Read the model definition and answer for the solid it produces. Units are mm, in the model's axes. Give positions to 0.01 mm unless a question says otherwise; leave off trailing zeros. Order: outer loops, then holes, each group sorted by start corner. A loop starts at its lowest first (then second) coordinate and runs counter-clockwise, first axis right, second up. Notation, with made-up numbers: (-9.75, 4.5) - (45.25, 4.5) arc R11 ccw to (45.25, 21.5) - close; hole circle Ø11 at (5.5, -2). An arc over 180 degrees is marked (long way). Write each question's results on one line, items separated by ' | '.
from build123d import *

# Parameters (mm, degrees)
BOSS_EXTRUDE1_DEPTH = 6.35
FILLET1_R           = 19.05
SKETCH4_R           = 10.5
SKETCH4_R_2         = 6.4
SKETCH4_R_3         = 1.5
CUT_EXTRUDE1_DEPTH  = 7.35


with BuildPart() as part:
    # Sketch3 → Boss-Extrude1 (new body)
    with BuildSketch(Plane.XY):
        Polygon((-152.4, 25.4), (50.8, 25.4), (175.63877155, -62.0130489), (-27.56122845, -62.0130489), align=None)
    extrude(amount=BOSS_EXTRUDE1_DEPTH)

    # Fillet1
    fillet1_edges = [part.edges().sort_by_distance(p)[0] for p in [
        (-152.4, 25.4, 3.175),
        (50.8, 25.4, 3.175),
        (175.63877155, -62.0130489, 3.175),
        (-27.56122845, -62.0130489, 3.175),
    ]]
    fillet(fillet1_edges, radius=FILLET1_R)

    # Sketch4 → Cut-Extrude1 (cut, through all)
    with BuildSketch(Plane.XY.offset(6.35)):
        with Locations((-91.981119015, 6.35)):
            Circle(SKETCH4_R)
        with Locations((38.393558072, 0)):
            Circle(SKETCH4_R_2)
        with Locations((-21.554786522, -42.9630489)):
            Circle(SKETCH4_R)
        with Locations((115.219890565, -42.9630489)):
            Circle(SKETCH4_R)
        with Locations((44.793558072, 14.117011015)):
            Circle(SKETCH4_R_3)
        with Locations((53.819248236, 1.515942923)):
            Circle(SKETCH4_R_3)
        with Locations((47.419248236, -12.601068092)):
            Circle(SKETCH4_R_3)
        with Locations((31.993558072, -14.117011015)):
            Circle(SKETCH4_R_3)
        with Locations((22.967867907, -1.515942923)):
            Circle(SKETCH4_R_3)
        with Locations((29.367867907, 12.601068092)):
            Circle(SKETCH4_R_3)
    extrude(amount=-CUT_EXTRUDE1_DEPTH, mode=Mode.SUBTRACT)


solid = part.part
(1) Section B-B (y = -50.5) is taken. Give the vertices of the cut face in (x, z), plus the area to 3 significant figures.
Conclusion:
outline: (-44, 0) - (-28.87, 0) - (-28.87, 6.35) - (-44, 6.35) - close; (-14.24, 0) - (107.91, 0) - (107.91, 6.35) - (-14.24, 6.35) - close; (122.53, 0) - (132.72, 0) - (132.72, 6.35) - (122.53, 6.35) - close | area: 936 mm^2
(2) Section A-A (z = 3.5) is taken. State how many separate pieces and enclosed holes the cut face has, plus the area to 3 significant figures.
Conclusion:
separate pieces: 1 | enclosed holes: 10 | area: 15,200 mm^2
(3) Section D-D (x = -42) is taken. Give the vertices of the cut face in (y, z), plus the area to 3 significant figures.
Conclusion:
outline: (-51.9, 0) - (25.4, 0) - (25.4, 6.35) - (-51.9, 6.35) - close | area: 491 mm^2
(4) Consider probe 1 along X at (y, z) = (-37, 1.5); probe 2 along X at (y, z) = (-41.5, 5.75); probe 3 along Y at (x, z) = (113, 6). Determine where each line is inside the solid, lowest interval first. Write a range as [from, to].
Conclusion:
probe 1: [-63.28, -30.2], [-12.91, 106.58], [123.86, 133.31] | probe 2: [-56.86, -31.95], [-11.16, 104.82], [125.62, 134.21] | probe 3: [-62.01, -53.23], [-32.7, -18.15]
(5) Section C-C (x = 41) is taken. Give the vertices of the cut face in (y, z).
Conclusion:
outline: (-62.01, 0) - (-5.85, 0) - (-5.85, 6.35) - (-62.01, 6.35) - close; (5.85, 0) - (25.4, 0) - (25.4, 6.35) - (5.85, 6.35) - close
(6) The mould has two halves that part along X. Classify faces 1 (the face through (13, -18, 6.35)), 2 (the face through (90.44, -2.356, 3.131)), 3 (the face through (-22.922, -32.552, 3.219)), 4 (the face through (33.31, -3.89, 3.22)): pulls with the +X half, pulls with the -X half, needs draft (parallel to the pull), parting line crosses it, or undercut.
Conclusion:
face 1: needs draft | face 2: pulls with the +X half | face 3: undercut | face 4: undercut
(7) This flat-tipped pin is pushed along its axis until it touches: pin 1 (2 mm diameter, centred on y = -29, z = 2.5, fed in from +X). Where does it stop, or does it pass through?
Conclusion:
pin 1: x = 129.18
